The model under review builds one solid part; all positions refer to its coordinate system, in mm. Coordinates: 2 decimals unless noted, no trailing zeros. Loops run counter-clockwise (first coordinate to the right, second up) from the corner with the lowest first, then second, coordinate; pieces in that order, holes last. Notation, with made-up numbers: (53, 17.5) - (63, 17.5) arc R11 ccw to (63, 33.5) - close; hole circle Ø3 at (62.25, 2.5). An arc over 180 degrees is marked (long way). Answer in a Markdown table with one row per item. Add a question column.
(1) For line 1 along Z through (x, y) = (59.5, 2.3); line 2 along X through (y, z) = (3.1, -29); line 3 along Z through (x, y) = (41, 1.45), list the stretches that pass through material, from the lowest coordinate up.
(2) We need section B-B on y = 3.8. Give the number of separate pieces and of enclosed holes in the cut face, plus the area to 3 significant figures.
(3) We need section A-A on x = 26. Write out the cut boundary in (y, z).
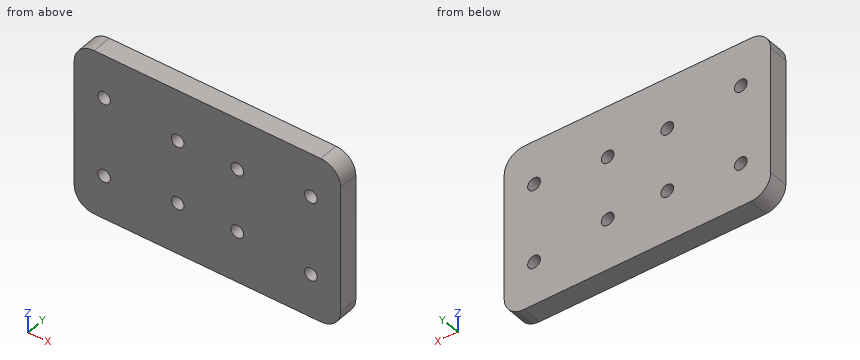
from build123d import *

# Parameters (mm, degrees)
SKETCH1_W           = 67
SKETCH1_H           = 42
SKETCH1_R           = 1.6
BOSS_EXTRUDE1_DEPTH = 5
SKETCH2_R           = 1.6
CUT_EXTRUDE1_DEPTH  = 6
FILLET1_R           = 5


with BuildPart() as part:
    # Sketch1 → Boss-Extrude1 (new body)
    with BuildSketch(Plane(origin=(0, 0, 0), x_dir=(1, 0, 0), z_dir=(0, 1, 0))):
        with Locations((33.5, 21)):
            Rectangle(SKETCH1_W, SKETCH1_H)
        with Locations((7.5, 31)):
            Circle(SKETCH1_R, mode=Mode.SUBTRACT)
        with Locations((7.5, 11)):
            Circle(SKETCH1_R, mode=Mode.SUBTRACT)
        with Locations((59.5, 11)):
            Circle(SKETCH1_R, mode=Mode.SUBTRACT)
        with Locations((59.5, 31)):
            Circle(SKETCH1_R, mode=Mode.SUBTRACT)
    extrude(amount=BOSS_EXTRUDE1_DEPTH)

    # Sketch2 → Cut-Extrude1 (cut, through all)
    with BuildSketch(Plane(origin=(0, 5, 0), x_dir=(1, 0, 0), z_dir=(0, 1, 0))):
        with Locations((41, 29)):
            Circle(SKETCH2_R)
        with Locations((41, 13)):
            Circle(SKETCH2_R)
        with Locations((26, 13)):
            Circle(SKETCH2_R)
        with Locations((26, 29)):
            Circle(SKETCH2_R)
    extrude(amount=-CUT_EXTRUDE1_DEPTH, mode=Mode.SUBTRACT)

    # Fillet1
    fillet1_edges = [part.edges().sort_by_distance(p)[0] for p in [
        (0, 2.5, -42),
        (67, 2.5, -42),
        (67, 2.5, 0),
        (0, 2.5, 0),
    ]]
    fillet(fillet1_edges, radius=FILLET1_R)


solid = part.part
Outcome:
| question | item | result |
|---|---|---|
| 1 | line 1 | -42 to -32.6, -29.4 to -12.6, -9.4 to 0 |
| 1 | line 2 | 0 to 24.4, 27.6 to 39.4, 42.6 to 67 |
| 1 | line 3 | -42 to -30.6, -27.4 to -14.6, -11.4 to 0 |
| 2 | separate pieces | 1 |
| 2 | enclosed holes | 8 |
| 2 | area | 2,730 mm² |
| 3 | outline | (0, -42) - (5, -42) - (5, -30.6) - (0, -30.6) - close; (0, -27.4) - (5, -27.4) - (5, -14.6) - (0, -14.6) - close; (0, -11.4) - (5, -11.4) - (5, 0) - (0, 0) - close |
